Design review of the part built by this model. Coordinates are the model's own, in mm. A direction names the side the tool comes from. Round coordinates to 2 decimals unless told otherwise and drop trailing zeros. Loops run counter-clockwise (first coordinate to the right, second up) from the corner with the lowest first, then second, coordinate; pieces in that order, holes last. Notation, with made-up numbers: (-29, 79.5) - (-8, 79.5) arc R24 cw to (-8, 102.5) - close; hole circle Ø9 at (72, 61). An arc over 180 degrees is marked (long way). Use one line per item in the form item = value. Start each with the question number.
(1) Wall thickness on probe 1 along Y at (x, z) = (298.45, 4.5) (3 decimals); probe 2 along X at (y, z) = (-185.5, 1): over which ranges is each line inside the solid? List them lowest first. Write a range as [from, to].
(2) We need section A-A, the plane y = -135. Write out the cut boundary in (x, z).
(3) Machinability: for faces 1 (the flat face through (14, -114.3, 6)), 2 (the flat face through (175, -113, 12.7)), which of the approach directions +Z, -Z, +X, -X, +Y, -Y give a long, thin tool a straight path to every point of the face, cutting with its end or side? Answer none if there is none.
(4) The part is to be moulded in two halves that separate along Y. For faces 3 (the flat face through (175, -113, 0)), 4 (the flat face through (175, -228.6, 6)), 5 (the flat face through (7.62, -178, 6)), say which applies: released by +Y, released by -Y, zero draft, split by the parting line, or undercut.
from build123d import *

# Parameters (mm, degrees)
SKETCH2_W           = 355.6
SKETCH2_H           = 228.6
BOSS_EXTRUDE1_DEPTH = 12.7
SKETCH3_R           = 3.175
CUT_EXTRUDE1_DEPTH  = 12.7
SKETCH4_W           = 12.7
SKETCH4_H           = 25.4
CUT_EXTRUDE2_DEPTH  = 13.7


with BuildPart() as part:
    # Sketch2 → Boss-Extrude1 (new body)
    with BuildSketch(Plane.XY):
        with Locations((177.8, -114.3)):
            Rectangle(SKETCH2_W, SKETCH2_H)
    extrude(amount=BOSS_EXTRUDE1_DEPTH)

    # Sketch3 → Cut-Extrude1 (cut)
    with BuildSketch(Plane.XY.offset(12.7)):
        with Locations((298.45, -114.3)):
            Circle(SKETCH3_R)
    extrude(amount=-CUT_EXTRUDE1_DEPTH, mode=Mode.SUBTRACT)

    # Sketch4 → Cut-Extrude2 (cut, through all)
    with BuildSketch(Plane.XY.offset(12.7)):
        with Locations((13.97, -76.2)):
            Rectangle(SKETCH4_W, SKETCH4_H)
        with Locations((13.97, -127)):
            Rectangle(SKETCH4_W, SKETCH4_H)
        with Locations((13.97, -177.8)):
            Rectangle(SKETCH4_W, SKETCH4_H)
    extrude(amount=-CUT_EXTRUDE2_DEPTH, mode=Mode.SUBTRACT)


solid = part.part
Data:
q1.probe_1 = [-228.6, -117.475], [-111.125, 0]
q1.probe_2 = [0, 7.62], [20.32, 355.6]
q2.outline = (0, 0) - (7.62, 0) - (7.62, 12.7) - (0, 12.7) - close; (20.32, 0) - (355.6, 0) - (355.6, 12.7) - (20.32, 12.7) - close
q3.face_1 = +Z, -Z
q3.face_2 = +Z, +X, -X, +Y, -Y
q4.face_3 = zero draft
q4.face_4 = released by -Y
q4.face_5 = undercut
